The model under review builds one solid part; all positions refer to its coordinate system, in mm. Face numbers are marked on the shaded views. A direction names the side the tool comes from. Coordinates: 2 decimals unless noted, no trailing zeros. Write each loop counter-clockwise with the first axis right and the second up, starting at its lowest first coordinate (ties: lowest second). Pieces come first, ordered by that corner, then holes. Notation, with made-up numbers: M 51,70.25 L 86,70.25 A18 ccw 86,74.25 Z; hole C -15,2.25 d1. An arc over 180 degrees is marked long. Answer as a JSON object with one key per item and string values.
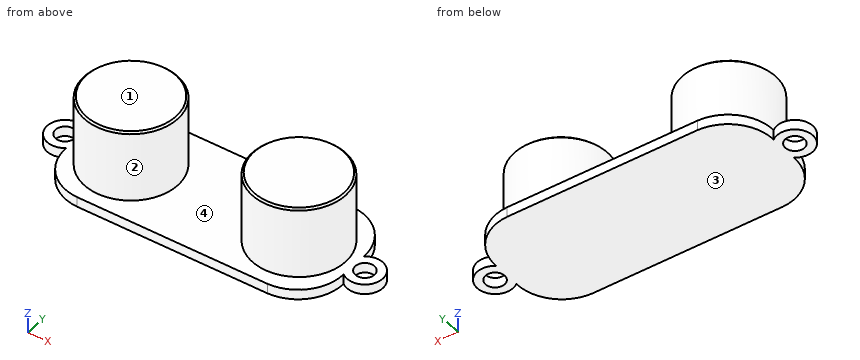
```python
from build123d import *

# Parameters (mm, degrees)
SKETCH007_R     = 1.6
PAD002_DEPTH    = 1.68
SKETCH008_R     = 7.8
PAD003_DEPTH    = 12
CHAMFER005_SIZE = 0.3


with BuildPart() as part:
    # Sketch007 → Pad002 (new body)
    with BuildSketch(Plane.XY):
        with BuildLine():
            Line((-15.86, -10), (15.86, -10))
            ThreePointArc((15.86, -10), (21.088323, -7.686238), (23.129445, -2.345574))
            ThreePointArc((23.129445, -2.345574), (28.000116, 0), (23.129445, 2.345574))
            ThreePointArc((23.129445, 2.345574), (21.088323, 7.686238), (15.86, 10))
            Line((-15.86, 10), (15.86, 10))
            ThreePointArc((-15.86, 10), (-21.088323, 7.686238), (-23.129445, 2.345574))
            ThreePointArc((-23.129445, 2.345574), (-28.000116, 0), (-23.129445, -2.345574))
            ThreePointArc((-23.129445, -2.345574), (-21.088323, -7.686238), (-15.86, -10))
        make_face()
        with Locations((-25, 0)):
            Circle(SKETCH007_R, mode=Mode.SUBTRACT)
        with Locations((25, 0)):
            Circle(SKETCH007_R, mode=Mode.SUBTRACT)
    extrude(amount=PAD002_DEPTH)

    # Sketch008 → Pad003 (new body)
    with BuildSketch(Plane.XY.offset(1.68)):
        with Locations((-14, 0)):
            Circle(SKETCH008_R)
        with Locations((14, 0)):
            Circle(SKETCH008_R)
    extrude(amount=PAD003_DEPTH)

    # Chamfer005
    chamfer005_edges = [part.edges().sort_by_distance(p)[0] for p in [
        (6.2, 0, 13.68),
        (-21.8, 0, 13.68),
    ]]
    chamfer(chamfer005_edges, length=CHAMFER005_SIZE)


solid = part.part
```
(1) For the marked faces 1 and 2, list the 3-axis set-ups (+Z, -Z, +X, -X, +Y, -Y) from which the entire face can be reached by the end or side of a thin tool; tool diameter is ignored.
Results list:
{"face 1": "+Z, +X, -X, +Y, -Y", "face 2": "+Z"}
(2) Add section A-A on x = -25. Give the boundary of the cut face in (y, z).
Results list:
{"outline": "M -3,0 L -1.6,0 L -1.6,1.68 L -3,1.68 Z; M 1.6,0 L 3,0 L 3,1.68 L 1.6,1.68 Z"}
(3) For pin 1 Ø3 at (y, z) = (1.5, 3.5) entering from -X; pin 2 Ø2 at (y, z) = (-2.5, 6) entering from -X; pin 3 Ø3 at (y, z) = (-1.5, 4) entering from +X; pin 4 Ø5 at (x, y) = (25, 0) entering from -Z, all flat-tipped, find the tip position at first contact; note any pin that passes through.
Results list:
{"pin 1": "x = -21.8", "pin 2": "x = -21.65", "pin 3": "x = 21.8", "pin 4": "z = 0"}
(4) Wall thickness on line 1 along Y through (x, z) = (25, 1.05); line 2 along Z through (x, y) = (7, 4); line 3 along X through (y, z) = (0.25, 12.75): over which ranges is each line inside the solid? List them lowest first. Write a range as from..to.
Results list:
{"line 1": "-3..-1.6, 1.6..3", "line 2": "0..1.68", "line 3": "-21.8..-6.2, 6.2..21.8"}
(5) Add section D-D on x = -14. Give the boundary of the cut face in (y, z), and give its area (3 significant figures).
Results list:
{"outline": "M -10,0 L 10,0 L 10,1.68 L 7.8,1.68 L 7.8,13.38 L 7.5,13.68 L -7.5,13.68 L -7.8,13.38 L -7.8,1.68 L -10,1.68 Z", "area": "221 mm²"}
(6) Add section B-B on y = 0. Give the boundary of the cut face in (x, z), and give its area (3 significant figures).
Results list:
{"outline": "M -28,0 L -26.6,0 L -26.6,1.68 L -28,1.68 Z; M -23.4,0 L 23.4,0 L 23.4,1.68 L 21.8,1.68 L 21.8,13.38 L 21.5,13.68 L 6.5,13.68 L 6.2,13.38 L 6.2,1.68 L -6.2,1.68 L -6.2,13.38 L -6.5,13.68 L -21.5,13.68 L -21.8,13.38 L -21.8,1.68 L -23.4,1.68 Z; M 26.6,0 L 28,0 L 28,1.68 L 26.6,1.68 Z", "area": "458 mm²"}
(7) Draft analysis for pull direction X (two halves, no side actions). For the marked faces 3 and 4, state which applies: released by +X, released by -X, zero draft, split by the parting line, or undercut.
Results list:
{"face 3": "zero draft", "face 4": "undercut"}
(8) Add section C-C on z = 1. Give the boundary of the cut face in (x, y).
Results list:
{"outline": "M -23.13,-2.35 A7.44 ccw -15.86,-10 L 15.86,-10 A7.44 ccw 23.13,-2.35 A3 ccw long 23.13,2.35 A7.44 ccw 15.86,10 L -15.86,10 A7.44 ccw -23.13,2.35 A3 ccw long Z; hole C -25,0 d3.2; hole C 25,0 d3.2"}
